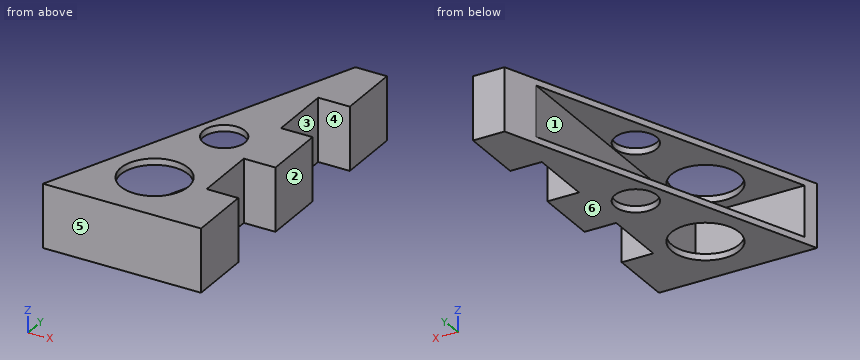
```python
from build123d import *

# Parameters (mm, degrees)
EXTRUDE_1_DEPTH     = 10
CUT_EXTRUDE_START   = 19.214766
SKETCH_3_W          = 8
SKETCH_3_H          = 48
CUT_EXTRUDE_4_DEPTH = 17.2
SKETCH_4_R          = 5.333163539
SKETCH_4_R_2        = 3.300328709
CUT_EXTRUDE_6_DEPTH = 67.968962262


with BuildPart() as part:
    # 草图1 → 凸台-拉伸1 (new body)
    with BuildSketch(Plane.XY):
        Polygon((38.414765995, 50), (18.414765995, 0), (43.414765995, 0), (43.414765995, 10), (38.414765995, 10), (38.414765995, 20), (43.414765995, 20), (43.414765995, 30), (38.414765995, 30), (38.414765995, 40), (43.414765995, 40), (43.414765995, 50), align=None)
    extrude(amount=-EXTRUDE_1_DEPTH)

    # 草图3 → 切除-拉伸4 (cut)
    with BuildSketch(Plane(origin=(0, 0, 0), x_dir=(0, 0, -1), z_dir=(1, 0, 0)).offset(CUT_EXTRUDE_START)):
        with Locations((5, 26)):
            Rectangle(SKETCH_3_W, SKETCH_3_H)
    extrude(amount=CUT_EXTRUDE_4_DEPTH, mode=Mode.SUBTRACT)

    # 草图4 → 切除-拉伸6 (cut, through all)
    with BuildSketch(Plane.XY):
        with Locations((30.601447123, 9.277555354)):
            Circle(SKETCH_4_R)
        with Locations((32.944682438, 24.013712258)):
            Circle(SKETCH_4_R_2)
    extrude(amount=-CUT_EXTRUDE_6_DEPTH, mode=Mode.SUBTRACT)


solid = part.part
```
The listing builds one solid part. Answer for the finished solid, in the listing's coordinates (mm). Face numbers are marked on the shaded views. A direction names the side the tool comes from. Give positions to 0.01 mm unless a question says otherwise; leave off trailing zeros. Loops run counter-clockwise (first coordinate to the right, second up) from the corner with the lowest first, then second, coordinate; pieces in that order, holes last. Notation, with made-up numbers: (88.25, 32.5) - (138.25, 32.5) arc R16 ccw to (138.25, 59.5) - close; hole circle Ø4 at (-3.75, 36.25). An arc over 180 degrees is marked (long way). Answer as CSV lines item,"result". Start each with the question number.
Item 1: A cutting plane is placed at C-C on z = -8.25. Determine the outline of the cut face in (x, y), then the cut area to 3 significant figures.
Item 2: A cutting plane is placed at B-B on y = 11. Determine the outline of the cut face in (x, z), then the cut area to 3 significant figures.
Item 3: Find the intervals of material crossed by line 1 (Y direction, x = 42.25, z = -5.75); line 2 (Z direction, x = 24.5, y = 14.5); line 3 (X direction, y = 14, z = -2.75), in increasing order. Write a range as from..to.
Item 4: A cutting plane is placed at D-D on x = 31. Determine the outline of the cut face in (y, z).
Item 5: The mould has two halves that part along Y. Classify the marked faces 4, 5 and 6: +Y half, -Y half, draft (parallel to the pull), parting line (faces both ways), or undercut.
Item 6: Each of these flat-tipped pins is pushed along its axis until it touches: pin 1 (1.5 mm diameter, centred on x = 29, z = -8, fed in from +Y); pin 2 (5 mm diameter, centred on x = 26, y = 21, fed in from -Z); pin 3 (3 mm diameter, centred on y = 5, z = -4.5, fed in from -X). Where does it stop, or does it pass through?
Item 7: A cutting plane is placed at A-A on x = 40.75. Determine the outline of the cut face in (y, z).
Item 8: For the marked faces 1, 2 and 3, determine the directions among +Z, -Z, +X, -X, +Y, -Y from which every point of the face is accessible in a straight line to the end or side of a thin tool.
Found:
1,outline,"(18.41, 0) - (43.41, 0) - (43.41, 10) - (38.41, 10) - (38.41, 20) - (43.41, 20) - (43.41, 30) - (38.41, 30) - (38.41, 40) - (43.41, 40) - (43.41, 50) - (38.41, 50) - (36.41, 45) - (36.41, 2) - (19.21, 2) - close"
1,area,"280 mm^2"
2,outline,"(22.81, -10) - (25.55, -10) - (25.55, -9) - (22.81, -9) - close; (22.81, -1) - (25.55, -1) - (25.55, 0) - (22.81, 0) - close; (35.65, -10) - (38.41, -10) - (38.41, 0) - (35.65, 0) - (35.65, -1) - (36.41, -1) - (36.41, -9) - (35.65, -9) - close"
2,area,"27.0 mm^2"
3,line 1,"y = 0..10, 20..30, 40..50"
3,line 2,"z = -10..-9, -1..0"
3,line 3,"x = 36.41..38.41"
4,outline,"(0, -10) - (3.96, -10) - (3.96, -9) - (2, -9) - (2, -1) - (3.96, -1) - (3.96, 0) - (0, 0) - close; (14.6, -10) - (21.35, -10) - (21.35, -9) - (14.6, -9) - close; (14.6, -1) - (21.35, -1) - (21.35, 0) - (14.6, 0) - close; (26.68, -10) - (31.46, -10) - (31.46, -9) - (26.68, -9) - close; (26.68, -1) - (31.46, -1) - (31.46, 0) - (26.68, 0) - close"
5,face 4,"undercut"
5,face 5,"-Y half"
5,face 6,"draft"
6,pin 1,"stops at y = 2"
6,pin 2,"stops at z = -10"
6,pin 3,"stops at x = 36.41"
7,outline,"(0, -10) - (10, -10) - (10, 0) - (0, 0) - close; (20, -10) - (30, -10) - (30, 0) - (20, 0) - close; (40, -10) - (50, -10) - (50, 0) - (40, 0) - close"
8,face 1,"-X, +Y"
8,face 2,"+Z, -Z, +X, +Y, -Y"
8,face 3,"+Z, -Z, +X"
